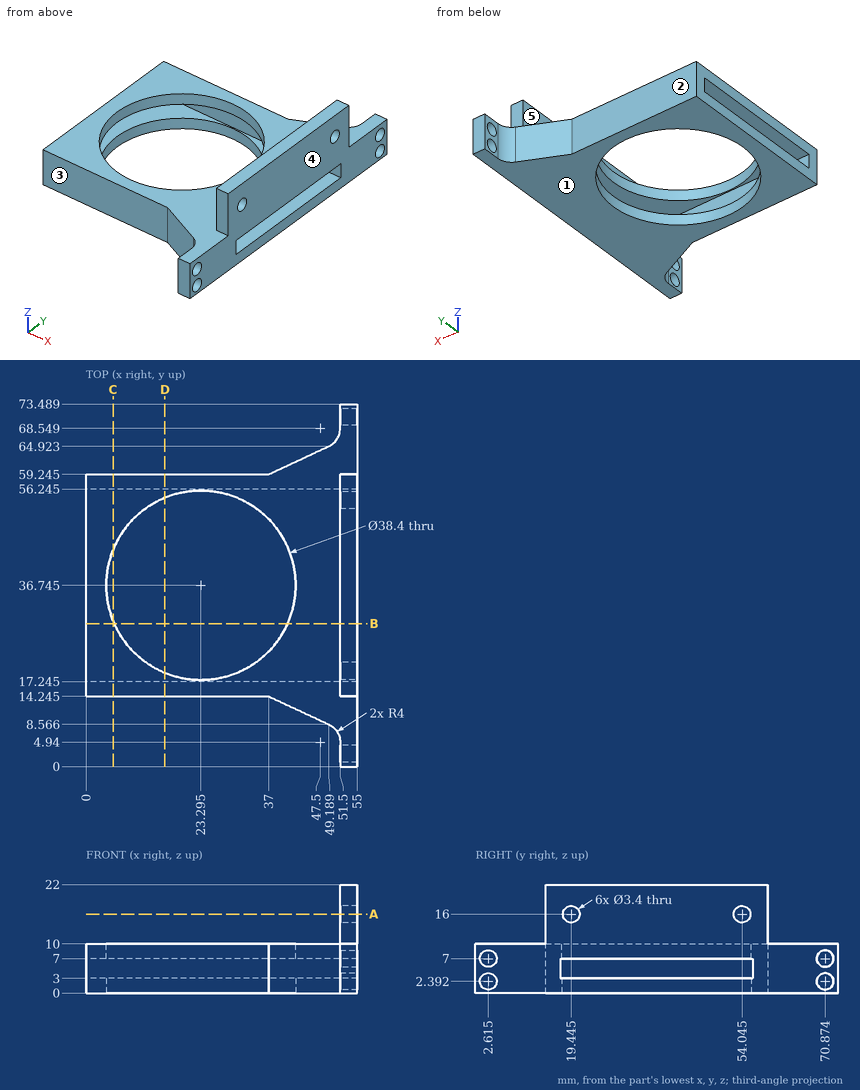
Study the drawing (mm; zero at the part's minimum x, y, z) and answer. A direction names the side the tool comes from. Give positions to 0.01 mm unless a question says otherwise; leave off trailing zeros. Write each loop counter-clockwise with the first axis right and the second up, starting at its lowest first coordinate (ties: lowest second). Pieces come first, ordered by that corner, then holes. Notation, with made-up numbers: (38.25, -33.75) -> (89.25, -33.75) arc R29 cw to (89.25, -13.75) -> close; hole circle Ø6 at (4, 59.25). An arc over 180 degrees is marked (long way). Write item = value, one per line. Start each with the question number.
1) Straight lines are drawn through the part: line 1 along Z through (x, y) = (25, 17.5); line 2 along Y through (x, z) = (13, 3.5) (1 decimal); line 3 along Z through (x, y) = (53, 43). For each, find the intervals that lie inside material, in ascending order.
2) The part is cut by section B-B, the plane y = 29. Determine the outline of the cut face in (x, z).
3) The part is cut by section D-D, the plane x = 16. Determine the outline of the cut face in (y, z) (1 decimal).
4) Each of these flat-tipped pins is pushed along its axis until it touches: pin 1 (11 mm diameter, centred on x = 11.5, z = 4.5, fed in from +Y) (1 decimal); pin 2 (1 mm diameter, centred on y = 39, z = 17.5, fed in from -X); pin 3 (12 mm diameter, centred on x = 13, y = 60.5, fed in from +Z). Where does it stop, or does it pass through?
5) The part is cut by section C-C, the plane x = 5.5. Determine the outline of the cut face in (y, z) (1 decimal).
6) The part is cut by section A-A, the plane z = 16. Determine the outline of the cut face in (x, y) (1 decimal).
7) Which of the six approach directions +Z, -Z, +X, -X, +Y, -Y give full straight-line access (tool end or side, diameter ignored) to the marked faces 1, 2, 3, 4 and 5?
Solutions:
q1.line_1 = 0 to 3, 7 to 10
q1.line_2 = 14.2 to 17.2, 56.2 to 59.2
q1.line_3 = 0 to 3, 7 to 22
q2.outline = (0, 0) -> (5.73, 0) -> (5.73, 3) -> (0, 3) -> close; (0, 7) -> (5.73, 7) -> (5.73, 10) -> (0, 10) -> close; (40.86, 0) -> (55, 0) -> (55, 3) -> (40.86, 3) -> close; (40.86, 7) -> (55, 7) -> (55, 22) -> (51.5, 22) -> (51.5, 10) -> (40.86, 10) -> close
q3.outline = (14.2, 0) -> (19, 0) -> (19, 3) -> (17.2, 3) -> (17.2, 7) -> (19, 7) -> (19, 10) -> (14.2, 10) -> close; (54.5, 0) -> (59.2, 0) -> (59.2, 10) -> (54.5, 10) -> (54.5, 7) -> (56.2, 7) -> (56.2, 3) -> (54.5, 3) -> close
q4.pin_1 = 59.2
q4.pin_2 = 51.5
q4.pin_3 = 10
q5.outline = (14.2, 0) -> (29.5, 0) -> (29.5, 3) -> (17.2, 3) -> (17.2, 7) -> (29.5, 7) -> (29.5, 10) -> (14.2, 10) -> close; (44, 0) -> (59.2, 0) -> (59.2, 10) -> (44, 10) -> (44, 7) -> (56.2, 7) -> (56.2, 3) -> (44, 3) -> close
q6.outline = (51.5, 14.2) -> (55, 14.2) -> (55, 17.7) -> (51.5, 17.7) -> close; (51.5, 21.1) -> (55, 21.1) -> (55, 52.3) -> (51.5, 52.3) -> close; (51.5, 55.7) -> (55, 55.7) -> (55, 59.2) -> (51.5, 59.2) -> close
q7.face_1 = -Z, +X, -X, +Y, -Y
q7.face_2 = +Z, -Z, -X, +Y
q7.face_3 = +Z, -Z, -X, -Y
q7.face_4 = +Z, -Z, +X, +Y, -Y
q7.face_5 = +Z, -X, +Y, -Y
